Verification items for the finished model (mm, model axes). A direction names the side the tool comes from. Round coordinates to 2 decimals unless told otherwise and drop trailing zeros. Order: outer loops, then holes, each group sorted by start corner. A loop starts at its lowest first (then second) coordinate and runs counter-clockwise, first axis right, second up. Notation, with made-up numbers: M 44.5,-16.5 L 83.5,-16.5 A24 cw 83.5,-4.5 Z; hole C 33.5,0.5 d7. An arc over 180 degrees is marked long. Return JSON: item names as keys, results as strings. Group by question number.
from build123d import *

# Parameters (mm, degrees)
BOSS_EXTRUDE1_DEPTH      = 152.4
BOSS_EXTRUDE1_DEPTH_BACK = 152.4
SKETCH3_R                = 6.35


with BuildPart() as part:
    # Sketch3 → Boss-Extrude1 (new, two sides: drawn at the far end of the back side and taken through both)
    with BuildSketch(Plane.XY.offset(-BOSS_EXTRUDE1_DEPTH_BACK)):
        Circle(SKETCH3_R)
    extrude(amount=BOSS_EXTRUDE1_DEPTH + BOSS_EXTRUDE1_DEPTH_BACK)

    # Sketch7 → 1/4-20 Tapped Hole1 (revolve, cut)
    with BuildSketch(Plane(origin=(0, 0, -152.4), x_dir=(0, 1, 0), z_dir=(1, 0, 0))):
        Polygon((0, 0), (0, 26.933816902), (2.5527, 25.4), (2.5527, 0), align=None)
    f_1_4_20_tapped_hole1 = revolve(axis=Axis((0, 0, -158.75), (0, 0, 1)), mode=Mode.SUBTRACT)

    # Mirror1: 1/4-20 Tapped Hole1 across plane
    add(f_1_4_20_tapped_hole1.mirror(Plane.XY), mode=Mode.SUBTRACT)


solid = part.part
1. Thickness scan on line 1 along Y through (x, z) = (0, -138.25); line 2 along X through (y, z) = (-3.5, 31); line 3 along X through (y, z) = (-1.5, -122). Record the ranges inside material, lowest first. Write a range as from..to.
2. Cross-section at A-A (z = 120.5). Enter the section's corners in (x, y).
3. Draft check along X on faces 3 (the face through (-0.767, 2.435, -139.878)), 4 (the face through (-1.38, -6.2, -2.13)), 5 (the face through (3, 0, 152.4)). Enter one of: +X half, -X half, draft (parallel to the pull), parting line (faces both ways), or undercut.
4. Access from +Z, -Z, +X, -X, +Y, -Y to the whole of each face (thin tool, end or side, straight path). Record for faces 1 (the face through (-0.767, 2.435, 139.878)), 2 (the face through (-0.13, 0.42, -125.73)).
5. Go/stop test with flat-tipped pins: pin 1 (5 mm diameter, centred on x = 3, z = -33.5, fed in from -Y); pin 2 (3 mm diameter, centred on x = 0, y = 0, fed in from -Z); pin 3 (3 mm diameter, centred on x = 0, y = 0, fed in from +Z). Record where each tip stops, or that it passes through.
Computed:
{
 "1": {"line 1": "y = -6.35..-2.55, 2.55..6.35", "line 2": "x = -5.3..5.3", "line 3": "x = -6.17..6.17"},
 "2": {"outline": "C 0,0 d12.7"},
 "3": {"face 3": "undercut", "face 4": "parting line", "face 5": "draft"},
 "4": {"face 1": "+Z", "face 2": "-Z"},
 "5": {"pin 1": "stops at y = -6.33", "pin 2": "stops at z = -126.37", "pin 3": "stops at z = 126.37"}
}
